```python
from build123d import *

# Parameters (mm, degrees)
SKETCH1_R           = 6
BOSS_EXTRUDE1_DEPTH = 1.3
SKETCH2_R           = 15
SKETCH2_R_2         = 1
BOSS_EXTRUDE2_DEPTH = 5
SKETCH3_R           = 2
CUT_EXTRUDE1_DEPTH  = 23.128940327
SKETCH4_R           = 3.75
CUT_EXTRUDE2_DEPTH  = 5.6


with BuildPart() as part:
    # Sketch1 → Boss-Extrude1 (new body)
    with BuildSketch(Plane(origin=(0, 0, 0), x_dir=(1, 0, 0), z_dir=(0, 1, 0))):
        with Locations(Location((0, 0, 0), (0, 0, 270))):
            Circle(SKETCH1_R)
    extrude(amount=BOSS_EXTRUDE1_DEPTH)

    # Sketch2 → Boss-Extrude2 (add)
    with BuildSketch(Plane(origin=(0, 1.3, 0), x_dir=(1, 0, 0), z_dir=(0, 1, 0))):
        with Locations(Location((0, 0, 0), (0, 0, 270))):
            Circle(SKETCH2_R)
        with Locations(Location((0, 12, 0), (0, 0, 270))):
            Circle(SKETCH2_R_2, mode=Mode.SUBTRACT)
        with Locations(Location((8.485281374, 8.485281374, 0), (0, 0, 270))):
            Circle(SKETCH2_R_2, mode=Mode.SUBTRACT)
        with Locations(Location((12, 0, 0), (0, 0, 270))):
            Circle(SKETCH2_R_2, mode=Mode.SUBTRACT)
        with Locations(Location((8.485281374, -8.485281374, 0), (0, 0, 270))):
            Circle(SKETCH2_R_2, mode=Mode.SUBTRACT)
        with Locations(Location((0, -12, 0), (0, 0, 270))):
            Circle(SKETCH2_R_2, mode=Mode.SUBTRACT)
        with Locations(Location((-8.485281374, -8.485281374, 0), (0, 0, 270))):
            Circle(SKETCH2_R_2, mode=Mode.SUBTRACT)
        with Locations(Location((-12, 0, 0), (0, 0, 270))):
            Circle(SKETCH2_R_2, mode=Mode.SUBTRACT)
        with Locations(Location((-8.485281374, 8.485281374, 0), (0, 0, 270))):
            Circle(SKETCH2_R_2, mode=Mode.SUBTRACT)
    extrude(amount=BOSS_EXTRUDE2_DEPTH)

    # Sketch3 → Cut-Extrude1 (cut, through all)
    with BuildSketch(Plane.XZ):
        with Locations(Location((0, 0, 0), (0, 0, 270))):
            Circle(SKETCH3_R)
    extrude(amount=-CUT_EXTRUDE1_DEPTH, mode=Mode.SUBTRACT)

    # Sketch4 → Cut-Extrude2 (cut)
    with BuildSketch(Plane(origin=(0, 6.3, 0), x_dir=(1, 0, 0), z_dir=(0, 1, 0))):
        with Locations(Location((0, 0, 0), (0, 0, 270))):
            Circle(SKETCH4_R)
    extrude(amount=-CUT_EXTRUDE2_DEPTH, mode=Mode.SUBTRACT)


solid = part.part
```
Here's how the part is built. I have some questions about the finished solid (model axes, mm). A direction names the side the tool comes from. Coordinates: 2 decimals unless noted, no trailing zeros. Order: outer loops, then holes, each group sorted by start corner. A loop starts at its lowest first (then second) coordinate and runs counter-clockwise, first axis right, second up.
1) Imagine slicing it at A-A on z = -12. List the corners of the cut face in (x, y) for me, and give its area (3 significant figures).
2) Imagine slicing it at D-D on y = 2. State how many separate pieces and enclosed holes the cut face has, and give its area (3 significant figures).
3) Which directions (+Z, -Z, +X, -X, +Y, -Y) give clear straight access to the entire face, cutting with the end or side of a thin tool? Please do faces 1 (the face through (0.165, 3.539, -3.746)), 2 (the face through (0.2, 1.3, 6.5)), 3 (the face through (-0.6, 3.8, -12.8)).
4) We'd pull the mould along Z, two halves only. Please class faces 4 (the face through (-3, 6.3, 3)), 5 (the face through (1.802, 0.641, 5.723)), 6 (the face through (-8.441, 3.765, 7.486)): +Z half, -Z half, draft (parallel to the pull), parting line (faces both ways), or undercut.
5) Will these pins go through, and if not, where does the flat tip stop? pin 1 (2 mm diameter, centred on y = 2, z = -11.5, fed in from +X); pin 2 (2.5 mm diameter, centred on x = 12, z = 0, fed in from -Y); pin 3 (3.5 mm diameter, centred on x = 0, z = 0, fed in from +Y).
6) Imagine slicing it at C-C on z = 0. List the corners of the cut face in (x, y) for me, and give its area (3 significant figures).
7) Imagine slicing it at B-B on x = 0. List the corners of the cut face in (y, z) for me.
8) I need wall thicknesses on line 1 (X direction, y = 3.3, z = 0); line 2 (X direction, y = 2.25, z = -7.75); line 3 (X direction, y = 3, z = -8). Which ranges of each line are inside material? Lowest first, please.
Response values:
1. outline: (-9, 1.3) - (-1, 1.3) - (-1, 6.3) - (-9, 6.3) - close; (1, 1.3) - (9, 1.3) - (9, 6.3) - (1, 6.3) - close
1. area: 80.0 mm2
2. separate pieces: 1
2. enclosed holes: 9
2. area: 638 mm2
3. face 1: +Y
3. face 2: -Y
3. face 3: +Y, -Y
4. face 4: draft
4. face 5: parting line
4. face 6: undercut
5. pin 1: stops at x = 10.71
5. pin 2: stops at y = 1.3
5. pin 3: passes through
6. outline: (-15, 1.3) - (-13, 1.3) - (-13, 6.3) - (-15, 6.3) - close; (-11, 1.3) - (-6, 1.3) - (-6, 0) - (-2, 0) - (-2, 0.7) - (-3.75, 0.7) - (-3.75, 6.3) - (-11, 6.3) - close; (2, 0) - (6, 0) - (6, 1.3) - (11, 1.3) - (11, 6.3) - (3.75, 6.3) - (3.75, 0.7) - (2, 0.7) - close; (13, 1.3) - (15, 1.3) - (15, 6.3) - (13, 6.3) - close
6. area: 101 mm2
7. outline: (0, -6) - (1.3, -6) - (1.3, -11) - (6.3, -11) - (6.3, -3.75) - (0.7, -3.75) - (0.7, -2) - (0, -2) - close; (0, 2) - (0.7, 2) - (0.7, 3.75) - (6.3, 3.75) - (6.3, 11) - (1.3, 11) - (1.3, 6) - (0, 6) - close; (1.3, -15) - (6.3, -15) - (6.3, -13) - (1.3, -13) - close; (1.3, 13) - (6.3, 13) - (6.3, 15) - (1.3, 15) - close
8. line 1: x = -15 to -13, -11 to -3.75, 3.75 to 11, 13 to 15
8. line 2: x = -12.84 to -9.16, -7.81 to 7.81, 9.16 to 12.84
8. line 3: x = -12.69 to -9.36, -7.61 to 7.61, 9.36 to 12.69
